The listing builds one solid part. Answer for the finished solid, in the listing's coordinates (mm). A direction names the side the tool comes from. Coordinates: 2 decimals unless noted, no trailing zeros. Order: outer loops, then holes, each group sorted by start corner. A loop starts at its lowest first (then second) coordinate and runs counter-clockwise, first axis right, second up. Notation, with made-up numbers: (25.5, 76) -> (45.5, 76) arc R31 ccw to (45.5, 111) -> close; hole circle Ø11 at (65.5, 46). An arc over 180 degrees is marked (long way). Write item = value, one per line. Start each with the question number.
```python
from build123d import *

# Parameters (mm, degrees)
BOSS_EXTRUDE1_DEPTH           = 3
BOSS_EXTRUDE1_TAPER           = 60
BOSS_EXTRUDE1_OTHER_WAY_DEPTH = 1
BOSS_EXTRUDE2_DEPTH           = 3
CUT_EXTRUDE1_DEPTH            = 7


with BuildPart() as part:
    # Sketch2 → Boss-Extrude1 (new body)
    with BuildSketch(Plane(origin=(0, 0, 0), x_dir=(1, 0, 0), z_dir=(0, 1, 0))):
        with BuildLine():
            Line((6.113925, -25.373803836), (43.9190025, -16.264511041))
            ThreePointArc((43.9190025, -16.264511041), (56.73, 0), (43.9190025, 16.264511041))
            Line((43.9190025, 16.264511041), (6.113925, 25.373803836))
            ThreePointArc((6.113925, 25.373803836), (-26.1, 0), (6.113925, -25.373803836))
        make_face()
    extrude(amount=BOSS_EXTRUDE1_DEPTH, taper=BOSS_EXTRUDE1_TAPER)

    # Sketch2 → Boss-Extrude1 other way (add)
    with BuildSketch(Plane(origin=(0, 0, 0), x_dir=(1, 0, 0), z_dir=(0, 1, 0))):
        with BuildLine():
            Line((6.113925, -25.373803836), (43.9190025, -16.264511041))
            ThreePointArc((43.9190025, -16.264511041), (56.73, 0), (43.9190025, 16.264511041))
            Line((43.9190025, 16.264511041), (6.113925, 25.373803836))
            ThreePointArc((6.113925, 25.373803836), (-26.1, 0), (6.113925, -25.373803836))
        make_face()
    extrude(amount=-BOSS_EXTRUDE1_OTHER_WAY_DEPTH)

    # Sketch1 → Boss-Extrude2 (add)
    with BuildSketch(Plane(origin=(0, 0, 0), x_dir=(1, 0, 0), z_dir=(0, 1, 0))):
        with BuildLine():
            Line((5.551725, 23.040580495), (43.3568025, 13.9312877))
            ThreePointArc((43.3568025, 13.9312877), (54.33, 0), (43.3568025, -13.9312877))
            Line((43.3568025, -13.9312877), (5.551725, -23.040580495))
            ThreePointArc((5.551725, -23.040580495), (-23.7, 0), (5.551725, 23.040580495))
        make_face()
    extrude(amount=-BOSS_EXTRUDE2_DEPTH)

    # Sketch3 → Cut-Extrude1 (cut, through all)
    with BuildSketch(Plane(origin=(0, 3, 0), x_dir=(1, 0, 0), z_dir=(0, 1, 0))):
        with BuildLine():
            Line((31.5, -3.5), (26.5, -3.5))
            ThreePointArc((26.5, -3.5), (23, 0), (26.5, 3.5))
            Line((26.5, 3.5), (31.5, 3.5))
            ThreePointArc((31.5, 3.5), (35, 0), (31.5, -3.5))
        make_face()
    extrude(amount=-CUT_EXTRUDE1_DEPTH, mode=Mode.SUBTRACT)


solid = part.part
```
Item 1: Each of these flat-tipped pins is pushed along its axis until it touches: pin 1 (1 mm diameter, centred on x = -17.5, y = -1, fed in from +Z); pin 2 (1.5 mm diameter, centred on y = 0.5, z = 4, fed in from +X); pin 3 (1.5 mm diameter, centred on x = 29, y = -1.5, fed in from -Z). Where does it stop, or does it pass through?
Item 2: For a pull along Z with two mould halves and no side action, classify faces 4 (the conical face through (51.784, 2.854, 0.22)), 5 (the flat face through (21.3, -1, -19.5)), 6 (the flat face through (29, 0, -3.5)) as pulls with the +Z half, pulls with the -Z half, needs draft (parallel to the pull), parting line crosses it, or undercut.
Item 3: Which of the six approach directions +Z, -Z, +X, -X, +Y, -Y give full straight-line access (tool end or side, diameter ignored) to faces 1 (the cylindrical face through (35, 0, 0)), 2 (the flat face through (24.19, -1.99, -18.55)), 3 (the cylindrical face through (-23.692, -1.986, 0.6))?
Item 4: Section A-A, the plane x = 0 is taken. Give the vertices of the cut face in (y, z).
Item 5: Consider probe 1 along X at (y, z) = (-1.75, -0.5); probe 2 along X at (y, z) = (-0.5, -7); probe 3 along Z at (x, y) = (14, -2.5). Determine where each line is inside the solid, lowest interval first.
A:
q1.pin_1 = 19.8
q1.pin_2 = 56.37
q1.pin_3 = -19.99
q2.face_4 = parting line crosses it
q2.face_5 = needs draft
q2.face_6 = undercut
q3.face_1 = +Y, -Y
q3.face_2 = -Z, +X, -Y
q3.face_3 = -Y
q4.outline = (-3, -23.7) -> (-1, -23.7) -> (-1, -26.1) -> (0, -26.1) -> (3, -20.9) -> (3, 20.9) -> (0, 26.1) -> (-1, 26.1) -> (-1, 23.7) -> (-3, 23.7) -> close
q5.probe_1 = -23.69 to 23.04, 34.96 to 54.32
q5.probe_2 = -25.14 to 55.2
q5.probe_3 = -21 to 21
